```python
from build123d import *

# Parameters (mm, degrees)
CROQUIS1_W              = 134
CROQUIS1_H              = 112
SALIENTE_EXTRUIR1_DEPTH = 3
CROQUIS2_W              = 52
CROQUIS2_H              = 92
SALIENTE_EXTRUIR2_DEPTH = 48.812
VACIADO1_T              = -5
CORTAR_EXTRUIR1_DEPTH   = 58.812
SALIENTE_EXTRUIR3_DEPTH = 48.812
CROQUIS5_W              = 58
CROQUIS5_H              = 40
SALIENTE_EXTRUIR4_DEPTH = 36
CROQUIS6_W              = 12
CROQUIS6_H              = 7.999587761
CORTAR_EXTRUIR2_DEPTH   = 58
CROQUIS7_R              = 1.5
CORTAR_EXTRUIR3_DEPTH   = 58
CROQUIS8_R              = 1.5
CORTAR_EXTRUIR4_DEPTH   = 58


with BuildPart() as part:
    # Croquis1 → Saliente-Extruir1 (new body)
    with BuildSketch(Plane.XY):
        Rectangle(CROQUIS1_W, CROQUIS1_H)
    extrude(amount=SALIENTE_EXTRUIR1_DEPTH)

    # Croquis2 → Saliente-Extruir2 (add)
    with BuildSketch(Plane.XY.offset(3)):
        with Locations((-21, -10)):
            Rectangle(CROQUIS2_W, CROQUIS2_H)
    extrude(amount=SALIENTE_EXTRUIR2_DEPTH)

    # Vaciado1
    vaciado1_openings = [part.faces().sort_by_distance(p)[0] for p in [
        (-21, -10, 51.812),
        (-18.128790187, -56, 23.864020885),
    ]]
    offset(amount=VACIADO1_T, openings=vaciado1_openings)

    # Croquis3 → Cortar-Extruir1 (cut)
    with BuildSketch(Plane.ZY.offset(47)):
        Polygon((15, -44), (15, -56), (51.812, -56), (51.812, 30.154), (44.811949005, 15.153963498), (43.00020398, 16.000146009), align=None)
    extrude(amount=-CORTAR_EXTRUIR1_DEPTH, mode=Mode.SUBTRACT)

    # Croquis4 → Saliente-Extruir3 (add)
    with BuildSketch(Plane.ZY.offset(47)):
        Polygon((43.00020398, 16.000146009), (44.811949005, 15.153963498), (51.812, 30.154), (50.004728246, 30.997397577), align=None)
    extrude(amount=-SALIENTE_EXTRUIR3_DEPTH)

    # Croquis5 → Saliente-Extruir4 (add)
    with BuildSketch(Plane.XY.offset(3)):
        with Locations((36, -36)):
            Rectangle(CROQUIS5_W, CROQUIS5_H)
    extrude(amount=SALIENTE_EXTRUIR4_DEPTH)

    # Croquis6 → Cortar-Extruir2 (cut)
    with BuildSketch(Plane(origin=(65, 0, 0), x_dir=(0, 0, -1), z_dir=(1, 0, 0))):
        with Locations((-33, -19.999793881)):
            Rectangle(CROQUIS6_W, CROQUIS6_H)
        Polygon((-39, -56), (-31, -56), (-39, -47.999587761), align=None)
    extrude(amount=-CORTAR_EXTRUIR2_DEPTH, mode=Mode.SUBTRACT)

    # Croquis7 → Cortar-Extruir3 (cut)
    with BuildSketch(Plane.XY.offset(5)):
        with Locations((-21, -46)):
            Circle(CROQUIS7_R)
        with Locations((-35, 46)):
            Circle(CROQUIS7_R)
        with Locations((55, 46)):
            Circle(CROQUIS7_R)
    extrude(amount=-CORTAR_EXTRUIR3_DEPTH, mode=Mode.SUBTRACT)

    # Croquis8 → Cortar-Extruir4 (cut)
    with BuildSketch(Plane(origin=(0, 36, 0), x_dir=(1, 0, 0), z_dir=(0, 1, 0))):
        with Locations(Location((-27, -31.812, 0), (0, 0, 270))):
            Circle(CROQUIS8_R)
        with Locations(Location((-12, -31.812, 0), (0, 0, 270))):
            Circle(CROQUIS8_R)
    extrude(amount=-CORTAR_EXTRUIR4_DEPTH, mode=Mode.SUBTRACT)


solid = part.part
```
The listing builds one solid part. Answer for the finished solid, in the listing's coordinates (mm). A direction names the side the tool comes from. Give positions to 0.01 mm unless a question says otherwise; leave off trailing zeros. Order: outer loops, then holes, each group sorted by start corner. A loop starts at its lowest first (then second) coordinate and runs counter-clockwise, first axis right, second up.
Item 1: Given pin 1 Ø14.5 at (y, z) = (-29.5, 21) entering from -X; pin 2 Ø13 at (x, z) = (28, 36) entering from +Y; pin 3 Ø2 at (x, z) = (30.5, 14) entering from +Y, each flat-ended and moving along its own axis, determine where each tip first touches the part or whether it passes through.
From the geometry:
pin 1: stops at x = -47
pin 2: stops at y = -24
pin 3: stops at y = -16
Item 2: Which of the six approach directions +Z, -Z, +X, -X, +Y, -Y give full straight-line access (tool end or side, diameter ignored) to faces 1 (the face through (7, -36, 21)), 2 (the face through (-21.325, -47.464, 2.535)), 3 (the face through (-21, 31, 28)), 4 (the face through (-21, -12, 5)), 5 (the face through (36, -24, 33))?
From the geometry:
face 1: +Z, +Y, -Y
face 2: +Z, -Z
face 3: none
face 4: -Y
face 5: +Z, +X, -X, +Y
Item 3: Find the intervals of material crossed by probe 1 along X at (y, z) = (-29, 8); probe 2 along Y at (x, z) = (55, 0.95); probe 3 along X at (y, z) = (10, 40), in increasing order.
From the geometry:
probe 1: x = -47 to -42, 0 to 5, 7 to 65
probe 2: y = -56 to 44.5, 47.5 to 56
probe 3: x = -47 to -42, 0 to 5
Item 4: The part is cut by section C-C, the plane z = 11. Give the vertices of the cut face in (x, y).
From the geometry:
outline: (-47, -56) - (-42, -56) - (-42, 31) - (0, 31) - (0, -56) - (5, -56) - (5, 36) - (-47, 36) - close; (7, -56) - (65, -56) - (65, -16) - (7, -16) - close
Item 5: The part is cut by section B-B, the plane x = 55. Give the vertices of the cut face in (y, z).
From the geometry:
outline: (-56, 0) - (44.5, 0) - (44.5, 3) - (-16, 3) - (-16, 27) - (-24, 27) - (-24, 39) - (-48, 39) - (-56, 31) - close; (47.5, 0) - (56, 0) - (56, 3) - (47.5, 3) - close
Item 6: For a pull along X with two mould halves and no side action, classify faces 6 (the face through (55.69, 44.67, 1.52)), 7 (the face through (36, -20, 27)) as pulls with the +X half, pulls with the -X half, needs draft (parallel to the pull), parting line crosses it, or undercut.
From the geometry:
face 6: undercut
face 7: needs draft
Item 7: The part is cut by section A-A, the plane y = -46. Give the vertices of the cut face in (x, z).
From the geometry:
outline: (-67, 0) - (-22.5, 0) - (-22.5, 5) - (-42, 5) - (-42, 15) - (-47, 15) - (-47, 3) - (-67, 3) - close; (-19.5, 0) - (67, 0) - (67, 3) - (65, 3) - (65, 39) - (7, 39) - (7, 3) - (5, 3) - (5, 15) - (0, 15) - (0, 5) - (-19.5, 5) - close
Item 8: The part is cut by section D-D, the plane y = 46. Give the vertices of the cut face in (x, z), and give its area (3 significant figures).
From the geometry:
outline: (-67, 0) - (-36.5, 0) - (-36.5, 3) - (-67, 3) - close; (-33.5, 0) - (53.5, 0) - (53.5, 3) - (-33.5, 3) - close; (56.5, 0) - (67, 0) - (67, 3) - (56.5, 3) - close
area: 384 mm2
